Autodesk Inventor part; units mm, degrees
ref_plane "YZ Plane" through (0, 0, 0) normal (1, 0, 0) x (0, 1, 0)
ref_plane "XZ Plane" through (0, 0, 0) normal (0, 1, 0) x (-1, 0, 0)
ref_plane "XY Plane" through (0, 0, 0) normal (0, 0, 1) x (1, 0, 0)
sketch "Skizze_Grundkörper" plane through (0, 0, 0) normal (0, 0, 1) x (1, 0, 0)
  line L0 (-63, 0) -> (63, 0)
  line L1 (0, -49) -> (0, 49)
  line L2 (45, -35) -> (-45, -35)
  line L3 (-45, -35) -> (-45, 35)
  line L4 (-45, 35) -> (45, 35)
  line L5 (45, 35) -> (45, -35)
  line L6 (45, -35) -> (-45, 35) construction
  line L7 (-45, -35) -> (45, 35) construction
  point P0 (0, 0)
  dimension "Länge" = 90
  dimension "Höhe" = 70
extrude "Grundkörper" add sketch "Skizze_Grundkörper" along normal blind 10
sketch "Skizze2" plane through (0, 0, 10) normal (0, 0, 1) x (1, 0, 0)
  line L0 (-45, -35) -> (45, -35)
  line L1 (45, -35) -> (45, 35)
  line L2 (45, 35) -> (-45, 35)
  line L3 (-45, 35) -> (-45, -35)
  line L4 (-63, 0) -> (63, 0)
  line L5 (0, -49) -> (0, 49)
  point P0 (0, 0)
  point P1 (0, 17)
  dimension "d4" = 52
hole "Bohrung_9,7_mm" at (0, 17, 10) direction (0, 0, -1) diameter 9.7 end through all
sketch "Skizze3" plane through (0, 0, 10) normal (0, 0, 1) x (1, 0, 0)
  circle A0 centre (0, 17) radius 4.85
  line L0 (-45, -35) -> (45, -35)
  line L1 (45, -35) -> (45, 35)
  line L2 (45, 35) -> (-45, 35)
  line L3 (-45, 35) -> (-45, -35)
  line L4 (-63, 0) -> (63, 0)
  line L5 (0, -49) -> (0, 49)
  point P0 (0, 0)
  point P1 (-35, -29)
  point P2 (35, -29)
  dimension "d12" = 70
  dimension "d13" = 6
hole "Bohrung_5,5_mm" at (-35, -29, 10) at (35, -29, 10) direction (0, 0, -1) diameter 5.5 end through all
chamfer "Fase_10_mm" distance 10 angle 45 2 edges at (-45, 35, 5) (45, 35, 5)
properties part number "Werkstück_C" material "Stahl, unlegiert"
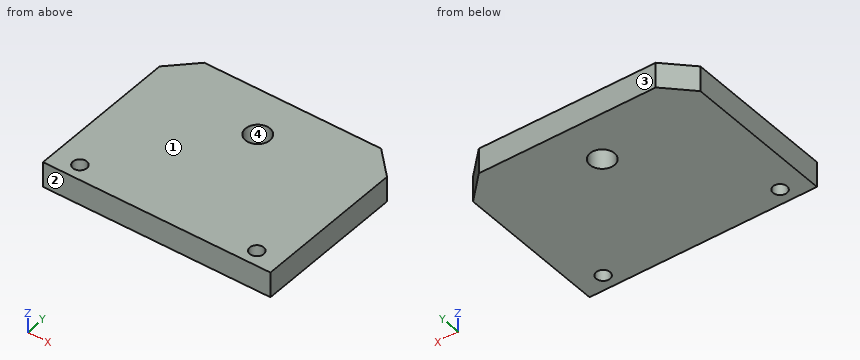
The model under review builds one solid part; all positions refer to its coordinate system, in mm. Face numbers are marked on the shaded views. Round coordinates to 2 decimals unless told otherwise and drop trailing zeros. Order: outer loops, then holes, each group sorted by start corner. A loop starts at its lowest first (then second) coordinate and runs counter-clockwise, first axis right, second up.
(1) Wall thickness on L1, parallel to X at y = -29, z = 7.5; L2, parallel to Y at x = 35, z = 6.75; L3, parallel to X at y = 17, z = 5.25: over which ranges is each line inside the solid? List them lowest first.
Working result:
L1: x = -45 to -37.75, -32.25 to 32.25, 37.75 to 45
L2: y = -35 to -31.75, -26.25 to 35
L3: x = -45 to -4.85, 4.85 to 45
(2) Mouldability with a two-part tool opening along Y and no side actions: class the marked faces 1, 2, 3 and 4 as released by +Y, released by -Y, zero draft, split by the parting line, or undercut.
Working result:
face 1: zero draft
face 2: released by -Y
face 3: released by +Y
face 4: undercut
(3) For P1, Ø1, axis at y = 26.5, z = 5, coming from the -X side; P2, Ø4.5, axis at x = 35, y = -29, coming from the -Z side, all flat-tipped, find the tip position at first contact; note any pin that passes through.
Working result:
P1: stops at x = -44
P2: passes through
(4) Take a section at B-B, the plane y = 17. State the section outline as (x, z) points.
Working result:
outline: (-45, 0) - (-4.85, 0) - (-4.85, 10) - (-45, 10) - close; (4.85, 0) - (45, 0) - (45, 10) - (4.85, 10) - close
(5) Take a section at A-A, the plane x = 0. State the section outline as (y, z) points, plus the area to 3 significant figures.
Working result:
outline: (-35, 0) - (12.15, 0) - (12.15, 10) - (-35, 10) - close; (21.85, 0) - (35, 0) - (35, 10) - (21.85, 10) - close
area: 603 mm2
(6) Take a section at C-C, the plane z = 6. State the section outline as (x, y) points, plus the area to 3 significant figures.
Working result:
outline: (-45, -35) - (45, -35) - (45, 25) - (35, 35) - (-35, 35) - (-45, 25) - close; hole circle Ø5.5 at (-35, -29); hole circle Ø9.7 at (0, 17); hole circle Ø5.5 at (35, -29)
area: 6,080 mm2
